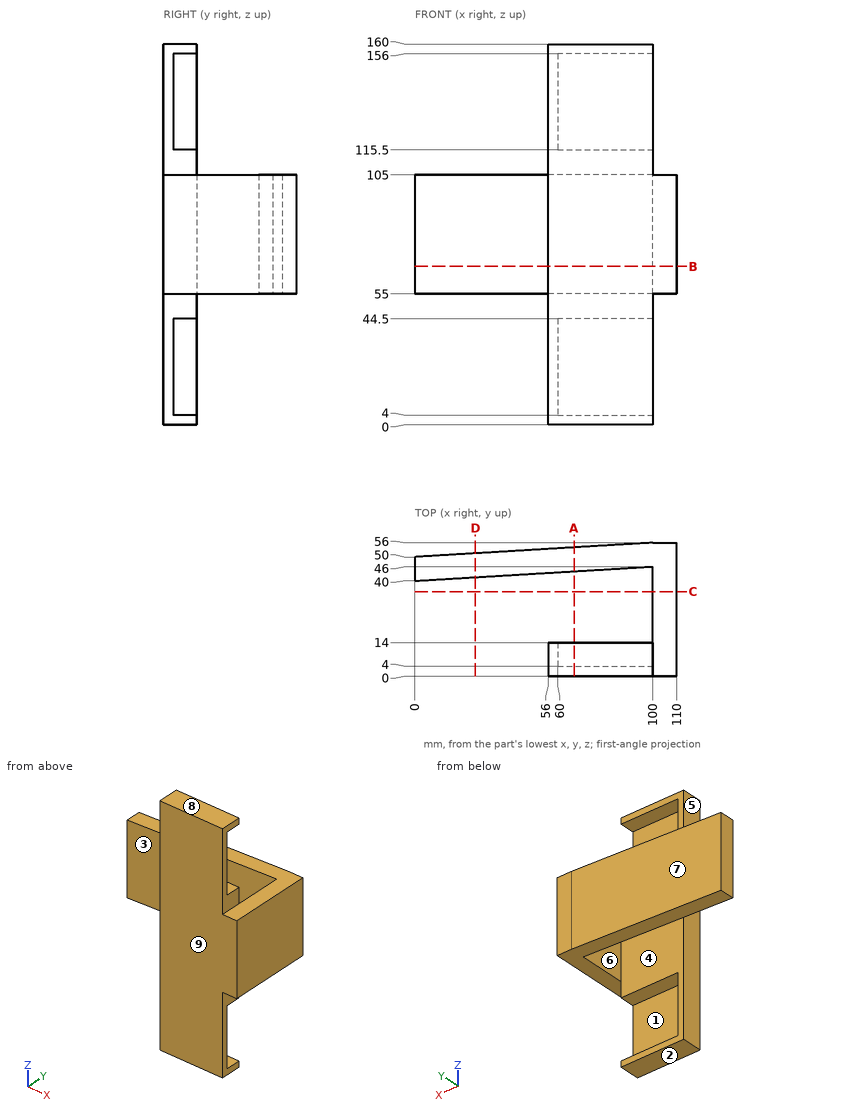
Geometry: see drawing. Coordinates: mm, zero at the bounding-box minimum. A direction names the side the tool comes from. Coordinates: 2 decimals unless noted, no trailing zeros. Loops run counter-clockwise (first coordinate to the right, second up) from the corner with the lowest first, then second, coordinate; pieces in that order, holes last.
(1) Material intervals for probe 1 along Z at (x, y) = (89, 7.5); probe 2 along Z at (x, y) = (15, 42); probe 3 along Y at (x, z) = (77.5, 43), sorted ascending.
(2) Set-up query: the marked faces 1, 2, 3, 4 and 5. Return all of +Z, -Z, +X, -X, +Y, -Y with unobstructed straight access to the full face (end or side cutting, diameter ignored); none if empty.
(3) Pull-direction query (Y, two-part tool) for the marked faces 6, 7, 8 and 9; classes: released by +Y, released by -Y, zero draft, split by the parting line, or undercut.
(4) First-contact query: pin 1 Ø4 at (y, z) = (5, 135) entering from +X; pin 2 Ø22 at (x, z) = (68.5, 52.5) entering from +Y; pin 3 Ø15.5 at (y, z) = (6, 108.5) entering from -X. Flat tips, straight axial feed; report the tip coordinate or a pass-through.
(5) Section B-B on z = 66.5. Return the cut outline in (x, y).
(6) Section D-D on x = 25.5. Return the cut outline in (y, z).
(7) Section A-A on x = 67. Return the cut outline in (y, z).
(8) Section C-C on y = 35.5. Return the cut outline in (x, z).
Data:
1. probe 1: z = 0 to 4, 44.5 to 115.5, 156 to 160
1. probe 2: z = 55 to 105
1. probe 3: y = 0 to 4
2. face 1: +X, +Y
2. face 2: -Z, +X, -X, +Y, -Y
2. face 3: +Z, -Z
2. face 4: +Z, -Z, -X
2. face 5: +Z, -Z, -X, -Y
3. face 6: undercut
3. face 7: released by +Y
3. face 8: zero draft
3. face 9: released by -Y
4. pin 1: stops at x = 100
4. pin 2: stops at y = 54.75
4. pin 3: stops at x = 56
5. outline: (0, 40) - (100, 46) - (100, 14) - (56, 14) - (56, 0) - (110, 0) - (110, 56) - (100, 56) - (0, 50) - close
6. outline: (41.53, 55) - (51.53, 55) - (51.53, 105) - (41.53, 105) - close
7. outline: (0, 0) - (14, 0) - (14, 4) - (4, 4) - (4, 44.5) - (14, 44.5) - (14, 115.5) - (4, 115.5) - (4, 156) - (14, 156) - (14, 160) - (0, 160) - close; (44.02, 55) - (54.02, 55) - (54.02, 105) - (44.02, 105) - close
8. outline: (100, 55) - (110, 55) - (110, 105) - (100, 105) - close
